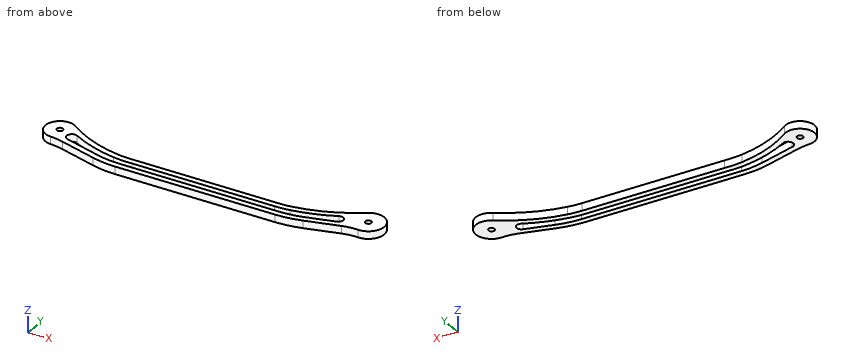
from build123d import *

# Parameters (mm, degrees)
SKETCH1_R           = 2.5
BOSS_EXTRUDE1_DEPTH = 6.2


with BuildPart() as part:
    # Sketch1 → Boss-Extrude1 (new body)
    with BuildSketch(Plane.XY):
        with BuildLine():
            ThreePointArc((-128.349445963, -11.974982784), (-122.593742509, -12.647675527), (-116.938372425, -13.911569107))
            Line((-116.938372425, -13.911569107), (-87, -22.25))
            ThreePointArc((-87, -22.25), (-77.031989093, -24.309319739), (-66.876941087, -25))
            Line((-66.876941087, -25), (65.326528755, -25))
            ThreePointArc((65.326528755, -25), (76.171142315, -24.268371831), (86.819214247, -22.086746937))
            Line((86.819214247, -22.086746937), (114.2908591, -14.5))
            ThreePointArc((114.2908591, -14.5), (120.491041615, -13.324280476), (126.8, -13.177230394))
            ThreePointArc((126.8, -13.177230394), (140.274563377, 3.600104754), (120, 10.810161116))
            ThreePointArc((120, 10.810161116), (96.313236011, -2.023267975), (70.328890052, -9.134769615))
            ThreePointArc((70.328890052, -9.134769615), (64.680941239, -9.783377892), (59, -10))
            Line((59, -10), (-59, -10))
            ThreePointArc((-59, -10), (-66.518658645, -9.998172905), (-74, -9.25))
            ThreePointArc((-74, -9.25), (-98.410939741, -2.539404949), (-120.554503776, 9.732051233))
            ThreePointArc((-120.554503776, 9.732051233), (-138.868880222, 4.055609252), (-128.349445963, -11.974982784))
        make_face()
        with BuildLine():
            Line((-85.658462739, -17.433333333), (-115.596835164, -9.09490244))
            ThreePointArc((-115.596835164, -9.09490244), (-118.701610917, -3.444269215), (-112.647605232, -1.22654437))
            ThreePointArc((-112.647605232, -1.22654437), (-94.281848906, -9.423130627), (-74.744170673, -14.194310873))
            ThreePointArc((-74.744170673, -14.194310873), (-66.831109196, -14.988771962), (-58.878274211, -15))
            Line((-58.878274211, -15), (59, -15))
            ThreePointArc((59, -15), (65.061701375, -14.768858984), (71.088199037, -14.076778302))
            ThreePointArc((71.088199037, -14.076778302), (88.608020432, -10.052780957), (105.35190821, -3.512221467))
            ThreePointArc((105.35190821, -3.512221467), (110.845938526, -5.730539831), (108.152661113, -11.007997765))
            Line((108.152661113, -11.007997765), (85.488206013, -17.26716012))
            ThreePointArc((85.488206013, -17.26716012), (75.499552441, -19.313680413), (65.326528755, -20))
            Line((65.326528755, -20), (-66.876941087, -20))
            ThreePointArc((-66.876941087, -20), (-76.354985893, -19.355365089), (-85.658462739, -17.433333333))
        make_face(mode=Mode.SUBTRACT)
        with Locations(Location((-127.574986581, 0, 0), (0, 0, 180))):
            Circle(SKETCH1_R, mode=Mode.SUBTRACT)
        with Locations(Location((127.574986581, 0, 0), (0, 0, 180))):
            Circle(SKETCH1_R, mode=Mode.SUBTRACT)
    extrude(amount=BOSS_EXTRUDE1_DEPTH)


solid = part.part
Read the model definition and answer for the solid it produces. Units are mm, in the model's axes. Give positions to 0.01 mm unless a question says otherwise; leave off trailing zeros. Write each loop counter-clockwise with the first axis right and the second up, starting at its lowest first coordinate (ties: lowest second). Pieces come first, ordered by that corner, then holes. Notation, with made-up numbers: (44.25, -17.5) - (77.25, -17.5) arc R12 ccw to (77.25, -11.5) - close; hole circle Ø8 at (67, 48). An arc over 180 degrees is marked (long way). Use CSV: the item, a comma, the result in double quotes. Start each with the question number.
(1) Find section C-C (z = 1). Give the vertices of the cut face in (x, y), plus the area to 3 significant figures.
(2) Consider line 1 along Y through (x, z) = (-25.5, 4.25); line 2 along X through (y, z) = (-2, 5.75); line 3 along X through (y, z) = (1, 3.25). Determine where each line is inside the solid, lowest interval first.
(3) Find section D-D (x = -107). Give the vertices of the cut face in (y, z).
(4) Find section B-B (y = -6.5). Give the vertices of the cut face in (x, z), plus the area to 3 significant figures.
(5) Find section A-A (x = 4.5). Give the vertices of the cut face in (y, z), plus the area to 3 significant figures.
(6) Given P1, Ø7.5, axis at x = -114.72, y = -4.94, coming from the -Z side; P2, Ø1, axis at x = 1.5, z = 1.5, coming from the +Y side; P3, Ø1.5, axis at y = -8.5, z = 1.5, coming from the -X side, each flat-ended and moving along its own axis, determine where each tip first touches the part or whether it passes through.
Findings below:
1,outline,"(-128.35, -11.97) arc R56 cw to (-116.94, -13.91) - (-87, -22.25) arc R75 ccw to (-66.88, -25) - (65.33, -25) arc R80.74 ccw to (86.82, -22.09) - (114.29, -14.5) arc R38.5 cw to (126.8, -13.18) arc R13.2 ccw (long way) to (120, 10.81) arc R117.7 cw to (70.33, -9.13) arc R74.6 cw to (59, -10) - (-59, -10) arc R75.65 cw to (-74, -9.25) arc R106.73 cw to (-120.55, 9.73) arc R12 ccw (long way) to start; hole circle Ø5 at (-127.57, 0); hole (-115.6, -9.09) - (-85.66, -17.43) arc R70 ccw to (-66.88, -20) - (65.33, -20) arc R75.74 ccw to (85.49, -17.27) - (108.15, -11.01) arc R4.02 ccw (long way) to (105.35, -3.51) arc R122.7 cw to (71.09, -14.08) arc R79.6 cw to (59, -15) - (-58.88, -15) arc R80.65 cw to (-74.74, -14.19) arc R111.73 cw to (-112.65, -1.23) arc R4.25 ccw (long way) to start; hole circle Ø5 at (127.57, 0)"
1,area,"3,430 mm2"
2,line 1,"-25 to -20, -15 to -10"
2,line 2,"-139.41 to -129.07, -126.07 to -117.79, -111.24 to -99.71, 96.37 to 126.07, 129.07 to 140.62"
2,line 3,"-139.53 to -129.87, -125.28 to -106.19, 103.2 to 125.28, 129.87 to 140.74"
3,outline,"(-16.68, 0) - (-11.49, 0) - (-11.49, 6.2) - (-16.68, 6.2) - close; (-4.18, 0) - (1.42, 0) - (1.42, 6.2) - (-4.18, 6.2) - close"
4,outline,"(-137.66, 0) - (-118.67, 0) - (-118.67, 6.2) - (-137.66, 6.2) - close; (-101.9, 0) - (-86.84, 0) - (-86.84, 6.2) - (-101.9, 6.2) - close; (82.88, 0) - (98.58, 0) - (98.58, 6.2) - (82.88, 6.2) - close; (111.05, 0) - (139.06, 0) - (139.06, 6.2) - (111.05, 6.2) - close"
4,area,"482 mm2"
5,outline,"(-25, 0) - (-20, 0) - (-20, 6.2) - (-25, 6.2) - close; (-15, 0) - (-10, 0) - (-10, 6.2) - (-15, 6.2) - close"
5,area,"62.0 mm2"
6,P1,"through"
6,P2,"y = -10"
6,P3,"x = -136.74"
